```python
from build123d import *

# Parameters (mm, degrees)
SKETCH1_W           = 60
SKETCH1_H           = 48
BOSS_EXTRUDE1_DEPTH = 13
SKETCH2_W           = 60
SKETCH2_H           = 48
BOSS_EXTRUDE2_DEPTH = 3
SKETCH3_W           = 54
SKETCH3_H           = 42
CUT_EXTRUDE1_DEPTH  = 13
CUT_EXTRUDE2_DEPTH  = 3
SKETCH5_W           = 30
SKETCH5_H           = 2
BOSS_EXTRUDE3_DEPTH = 10
CUT_EXTRUDE3_DEPTH  = 64.198101237
CUT_EXTRUDE4_DEPTH  = 10
CUT_EXTRUDE5_DEPTH  = 10
FILLET1_R           = 0.5


with BuildPart() as part:
    # Sketch1 → Boss-Extrude1 (new body)
    with BuildSketch(Plane(origin=(0, 0, 0), x_dir=(1, 0, 0), z_dir=(0, 1, 0))):
        Rectangle(SKETCH1_W, SKETCH1_H)
    extrude(amount=BOSS_EXTRUDE1_DEPTH)

    # Sketch2 → Boss-Extrude2 (add)
    with BuildSketch(Plane.XZ):
        Rectangle(SKETCH2_W, SKETCH2_H)
    extrude(amount=BOSS_EXTRUDE2_DEPTH)

    # Sketch3 → Cut-Extrude1 (cut)
    with BuildSketch(Plane(origin=(0, 13, 0), x_dir=(1, 0, 0), z_dir=(0, 1, 0))):
        Rectangle(SKETCH3_W, SKETCH3_H)
    extrude(amount=-CUT_EXTRUDE1_DEPTH, mode=Mode.SUBTRACT)

    # Sketch4 → Cut-Extrude2 (cut)
    with BuildSketch(Plane(origin=(27, 0, 39), x_dir=(0, 0, 1), z_dir=(-1, 0, 0))):
        with BuildLine():
            Line((-37.5, 3), (-37.5, 13))
            Line((-37.5, 13), (-33.5, 13))
            Line((-33.5, 13), (-33.5, 3))
            ThreePointArc((-33.5, 3), (-35.5, 1), (-37.5, 3))
        make_face()
        with BuildLine():
            Line((-40.5, 3), (-40.5, 13))
            Line((-40.5, 13), (-44.5, 13))
            Line((-44.5, 13), (-44.5, 3))
            ThreePointArc((-44.5, 3), (-42.5, 1), (-40.5, 3))
        make_face()
    extrude(amount=-CUT_EXTRUDE2_DEPTH, mode=Mode.SUBTRACT)

    # Sketch5 → Boss-Extrude3 (add)
    with BuildSketch(Plane(origin=(0, 0, 0), x_dir=(1, 0, 0), z_dir=(0, 1, 0))):
        with Locations((-12, 0)):
            Rectangle(SKETCH5_W, SKETCH5_H)
    extrude(amount=BOSS_EXTRUDE3_DEPTH)

    # Sketch6 → Cut-Extrude3 (cut, through all)
    with BuildSketch(Plane(origin=(-27, 0, 0), x_dir=(0, 0, -1), z_dir=(1, 0, 0))):
        with BuildLine():
            Line((-13, 3), (-13, 13))
            Line((-13, 13), (-9, 13))
            Line((-9, 13), (-9, 3))
            ThreePointArc((-9, 3), (-11, 1), (-13, 3))
        make_face()
    cut_extrude3 = extrude(amount=-CUT_EXTRUDE3_DEPTH, mode=Mode.SUBTRACT)

    # Mirror1: Cut-Extrude3 across plane
    add(cut_extrude3.mirror(Plane.XY), mode=Mode.SUBTRACT)

    # Sketch7 → Cut-Extrude4 (cut)
    with BuildSketch(Plane(origin=(0, 0, 21), x_dir=(-1, 0, 0), z_dir=(0, 0, -1))):
        with BuildLine():
            Line((-14, 3), (-14, 13))
            Line((-14, 13), (-10, 13))
            Line((-10, 13), (-10, 3))
            ThreePointArc((-10, 3), (-12, 1), (-14, 3))
        make_face()
        with BuildLine():
            Line((-17, 3), (-17, 13))
            Line((-17, 13), (-21, 13))
            Line((-21, 13), (-21, 3))
            ThreePointArc((-21, 3), (-19, 1), (-17, 3))
        make_face()
    extrude(amount=-CUT_EXTRUDE4_DEPTH, mode=Mode.SUBTRACT)

    # Sketch11 → Cut-Extrude5 (cut)
    with BuildSketch(Plane(origin=(0, 0, 0), x_dir=(1, 0, 0), z_dir=(0, 1, 0))):
        with BuildLine():
            Line((-20, 5), (20, 5))
            ThreePointArc((20, 5), (21.5, 6.5), (20, 8))
            Line((20, 8), (-20, 8))
            ThreePointArc((-20, 8), (-21.5, 6.5), (-20, 5))
        make_face()
        with BuildLine():
            Line((-20, 14), (20, 14))
            ThreePointArc((20, 14), (21.5, 15.5), (20, 17))
            Line((20, 17), (-20, 17))
            ThreePointArc((-20, 17), (-21.5, 15.5), (-20, 14))
        make_face()
        with BuildLine():
            Line((-20, -5), (20, -5))
            ThreePointArc((20, -5), (21.5, -6.5), (20, -8))
            Line((20, -8), (-20, -8))
            ThreePointArc((-20, -8), (-21.5, -6.5), (-20, -5))
        make_face()
        with BuildLine():
            Line((-20, -17), (20, -17))
            ThreePointArc((20, -17), (21.5, -15.5), (20, -14))
            Line((20, -14), (-20, -14))
            ThreePointArc((-20, -14), (-21.5, -15.5), (-20, -17))
        make_face()
    extrude(amount=-CUT_EXTRUDE5_DEPTH, mode=Mode.SUBTRACT)

    # Fillet1
    fillet1_edges = [part.edges().sort_by_distance(p)[0] for p in [
        (0, -3, 17),
        (21.5, -3, 15.5),
        (0, -3, 14),
        (-21.5, -3, 15.5),
        (0, -3, -5),
        (21.5, -3, -6.5),
        (0, -3, -8),
        (-21.5, -3, -6.5),
        (0, -3, 8),
        (21.5, -3, 6.5),
        (0, -3, 5),
        (-21.5, -3, 6.5),
        (-30, -3, 0),
        (0, -3, -17),
        (-21.5, -3, -15.5),
        (0, -3, -14),
        (21.5, -3, -15.5),
        (0, -3, -24),
        (30, -3, 0),
        (0, -3, 24),
        (-27, 6.5, 21),
        (-27, 6.5, -21),
        (27, 6.5, -21),
        (27, 6.5, 21),
        (-27, 5, -1),
        (-27, 5, 1),
        (3, 5, 1),
        (3, 5, -1),
        (-30, 5, -24),
        (30, 5, -24),
        (30, 5, 24),
        (-30, 5, 24),
    ]]
    fillet(fillet1_edges, radius=FILLET1_R)


solid = part.part
```
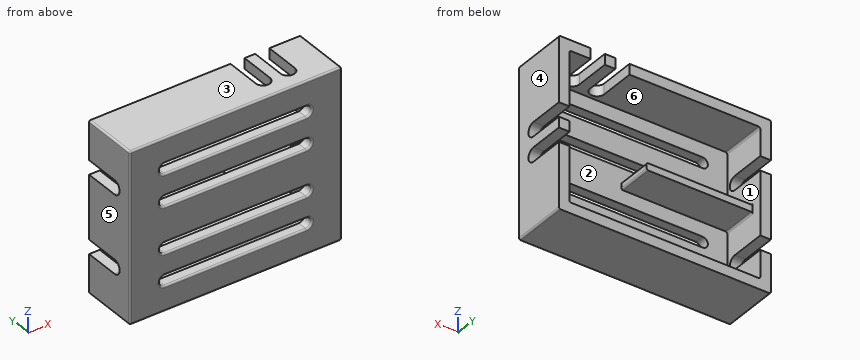
Verification items for the finished model (mm, model axes). Face numbers are marked on the shaded views. A direction names the side the tool comes from. Coordinates: 2 decimals unless noted, no trailing zeros. Write each loop counter-clockwise with the first axis right and the second up, starting at its lowest first coordinate (ties: lowest second). Pieces come first, ordered by that corner, then holes. Notation, with made-up numbers: (32, -25.5) - (88, -25.5) arc R21 cw to (88, -6.5) - close; hole circle Ø7 at (67, -20.5). An arc over 180 degrees is marked (long way). Write item = value, one per line.
Q1. Go/stop test with a flat-tipped pin: pin 1 Ø6 at (x, z) = (-10.5, 9.5) entering from +Y. Record where the tip stops, or that it passes through.
Answer:
pin_1 = 0
Q2. Access from +Z, -Z, +X, -X, +Y, -Y to the whole of each face (thin tool, end or side, straight path). Record for the marked faces 5 and 6.
Answer:
face_5 = +Z, -Z, -X, +Y, -Y
face_6 = +Y
Q3. Mould release check, pull along Z, two halves, no side actions. Record for the marked faces 1, 2, 3 and 4: released by +Z, released by -Z, zero draft, split by the parting line, or undercut.
Answer:
face_1 = undercut
face_2 = undercut
face_3 = released by +Z
face_4 = zero draft
Q4. Cross-section at C-C (z = -19). Enter the section's corners in (x, y).
Answer:
outline = (-30, -2.5) arc R0.5 ccw to (-29.5, -3) - (29.5, -3) arc R0.5 ccw to (30, -2.5) - (30, 13) - (27, 13) - (27, 0) - (-27, 0) - (-27, 13) - (-30, 13) - close
Q5. Cross-section at D-D (y = 4). Give the number of separate pieces and of enclosed holes in the cut face, plus the area to 3 significant figures.
Answer:
separate_pieces = 6
enclosed_holes = 0
area = 600 mm²
Q6. Cross-section at B-B (x = 24). Enter the section's corners in (y, z), plus the area to 3 significant figures.
Answer:
outline = (-3, -23.5) arc R0.5 ccw to (-2.5, -24) - (13, -24) - (13, -21) - (0, -21) - (0, 21) - (13, 21) - (13, 24) - (-2.5, 24) arc R0.5 ccw to (-3, 23.5) - close
area = 222 mm²
Q7. Material ranges on L1, parallel to Z at x = -10, y = 7.25; L2, parallel to X at y = 10, z = -8; L3, parallel to Z at x = 7, y = 2.5, recorded low to high. Write a range as from..to.
Answer:
L1 = -24..-21, -1..1, 21..24
L2 = -30..-27, 27..30
L3 = -24..-21, 21..24
Q8. Cross-section at A-A (z = 15.5). Enter the section's corners in (x, y), plus the area to 3 significant figures.
Answer:
outline = (-30, -2.5) arc R0.5 ccw to (-29.5, -3) - (-22, -3) arc R0.5 ccw to (-21.5, -2.5) - (-21.5, 0) - (-27, 0) - (-27, 13) - (-30, 13) - close; (21.5, -2.5) arc R0.5 ccw to (22, -3) - (29.5, -3) arc R0.5 ccw to (30, -2.5) - (30, 13) - (27, 13) - (27, 0) - (21.5, 0) - close
area = 129 mm²
